```python
from build123d import *

# Parameters (mm, degrees)
F3_R      = 4.7
F4_DEPTH  = 43
F8_DEPTH  = 43
F6_R      = 4.7
F6_R_2    = 4
F9_DEPTH  = 25
F7_R      = 4.7
F7_R_2    = 4
F10_DEPTH = 12
F11_R     = 2.75
F12_DEPTH = 4.701


# Not quite as in the source:
# - ends of sketch curves that miss each other by under 0.0002 mm in the source are joined


with BuildPart() as f4:
    # F3 (on Front) → F4 (new body)
    with BuildSketch(Plane.XZ):
        Circle(F3_R)
    extrude(amount=F4_DEPTH)

    # F5 (on face) → F8 (cut, through all)
    with BuildSketch(Plane.XZ.offset(43)):
        with BuildLine():
            Line((-1.25, -3.8), (0, -3.8))
            Line((0, -3.8), (1.25, -3.8))
            Line((1.25, -3.8), (1.25, -3.7))
            ThreePointArc((1.25, -3.7), (1.3085786438, -3.5585786438), (1.45, -3.5))
            Line((1.45, -3.5), (2, -3.5))
            Line((2, -3.5), (2, -3.05))
            ThreePointArc((2, -3.05), (2.0585786438, -2.9085786438), (2.2, -2.85))
            Line((2.2, -2.85), (3.15, -2.85))
            Line((3.15, -2.85), (3.15, -2.15))
            Line((3.15, -2.15), (2.2, -2.15))
            ThreePointArc((2.2, -2.15), (2.0585786438, -2.0914213562), (2, -1.95))
            Line((2, -1.95), (2, -1.887459))
            ThreePointArc((2, -1.887459), (2.1033535752, -1.771554046), (2.2, -1.65))
            Line((2.2, -1.65), (3.75, -1.65))
            Line((3.75, -1.65), (3.75, 0))
            Line((3.75, 0), (3.75, 1.65))
            Line((3.75, 1.65), (2.2, 1.65))
            ThreePointArc((2.2, 1.65), (2.1033535752, 1.771554046), (1.9999998047, 1.8874588157))
            Line((1.9999998047, 1.8874588157), (2, 1.95))
            ThreePointArc((2, 1.95), (2.0585786438, 2.0914213562), (2.2, 2.15))
            Line((2.2, 2.15), (3.15, 2.15))
            Line((3.15, 2.15), (3.15, 2.85))
            Line((3.15, 2.85), (2.2, 2.85))
            ThreePointArc((2.2, 2.85), (2.0585786438, 2.9085786438), (2, 3.05))
            Line((2, 3.05), (2, 3.5))
            Line((2, 3.5), (1.45, 3.5))
            ThreePointArc((1.45, 3.5), (1.3085786438, 3.5585786438), (1.25, 3.7))
            Line((1.25, 3.7), (1.25, 3.8))
            Line((1.25, 3.8), (0, 3.8))
            Line((0, 3.8), (-1.25, 3.8))
            Line((-1.25, 3.8), (-1.25, 3.7))
            ThreePointArc((-1.25, 3.7), (-1.3085786438, 3.5585786438), (-1.45, 3.5))
            Line((-1.45, 3.5), (-2, 3.5))
            Line((-2, 3.5), (-2, 3.05))
            ThreePointArc((-2, 3.05), (-2.0585786438, 2.9085786438), (-2.2, 2.85))
            Line((-2.2, 2.85), (-3.15, 2.85))
            Line((-3.15, 2.85), (-3.15, 2.15))
            Line((-3.15, 2.15), (-2.2, 2.15))
            ThreePointArc((-2.2, 2.15), (-2.0585786438, 2.0914213562), (-2, 1.95))
            Line((-2, 1.95), (-2, 1.887459))
            ThreePointArc((-2, 1.887459), (-2.1033535752, 1.771554046), (-2.2, 1.65))
            Line((-2.2, 1.65), (-3.75, 1.65))
            Line((-3.75, 1.65), (-3.75, 0))
            Line((-3.75, 0), (-3.75, -1.65))
            Line((-3.75, -1.65), (-2.2, -1.65))
            ThreePointArc((-2.2, -1.65), (-2.1033535752, -1.771554046), (-1.9999998047, -1.8874588157))
            Line((-1.9999998047, -1.8874588157), (-2, -1.95))
            ThreePointArc((-2, -1.95), (-2.0585786438, -2.0914213562), (-2.2, -2.15))
            Line((-2.2, -2.15), (-3.15, -2.15))
            Line((-3.15, -2.15), (-3.15, -2.85))
            Line((-3.15, -2.85), (-2.2, -2.85))
            ThreePointArc((-2.2, -2.85), (-2.0585786438, -2.9085786438), (-2, -3.05))
            Line((-2, -3.05), (-2, -3.5))
            Line((-2, -3.5), (-1.45, -3.5))
            ThreePointArc((-1.45, -3.5), (-1.3085786438, -3.5585786438), (-1.25, -3.7))
            Line((-1.25, -3.7), (-1.25, -3.8))
        make_face()
    extrude(amount=-F8_DEPTH, mode=Mode.SUBTRACT)

    # F6 (on face) → F9 (join)
    with BuildSketch(Plane.XZ.offset(43)):
        Circle(F6_R)
        Circle(F6_R_2, mode=Mode.SUBTRACT)
    extrude(amount=F9_DEPTH)

    # F7 (on face) → F10 (join)
    with BuildSketch(Plane(origin=(0, 0, 0), x_dir=(-1, 0, 0), z_dir=(0, 1, 0))):
        Circle(F7_R)
        Circle(F7_R_2, mode=Mode.SUBTRACT)
    extrude(amount=F10_DEPTH)

    # F11 (on Right) → F12 (cut, through all)
    with BuildSketch(Plane.YZ):
        with Locations((-62, 0)):
            Circle(F11_R)
    extrude(amount=-F12_DEPTH, mode=Mode.SUBTRACT)


solid = f4.part
```
The listing builds one solid part. Answer for the finished solid, in the listing's coordinates (mm). A direction names the side the tool comes from. Coordinates: 2 decimals unless noted, no trailing zeros. Write each loop counter-clockwise with the first axis right and the second up, starting at its lowest first coordinate (ties: lowest second). Pieces come first, ordered by that corner, then holes. Notation, with made-up numbers: (-2, -33) - (31, -33) arc R21 cw to (31, -14) - close; hole circle Ø10 at (53, 29.25). An arc over 180 degrees is marked (long way). Return JSON: item names as keys, results as strings. Group by question number.
1. Which of the six approach directions +Z, -Z, +X, -X, +Y, -Y give full straight-line access (tool end or side, diameter ignored) to faces 3 (the cylindrical face through (0.867, 5.916, -3.905)), 4 (the flat face through (0, -22, -3.8)), 5 (the flat face through (3.75, -22, 0)), 6 (the cylindrical face through (3.815, -55.325, 1.201)), 7 (the cylindrical face through (-4.19, -59.38, 0.83))?
2. A cutting plane is placed at A-A, the plane x = 0. Determine the outline of the cut face in (y, z), plus the area to 3 significant figures.
3. Straight lines are drawn through the part: L1, parallel to Z at x = 3.5, y = 6; L2, parallel to X at y = -27.5, z = -2.75; L3, parallel to Z at x = 0, y = 7. For each, find the intervals that lie inside material, in ascending order.
4. A cutting plane is placed at B-B, the plane z = 0. Determine the outline of the cut face in (x, y), plus the area to 3 significant figures.
5. Determine the mould class of faces 1 (the flat face through (-3, -22, 1.65)), 2 (the flat face through (-2, 12, 4)) for opening direction Z: released by +Z, released by -Z, zero draft, split by the parting line, or undercut.
6. Given pin 1 (1 mm diameter, centred on x = 3, y = -25.5, fed in from +Z); pin 2 (4 mm diameter, centred on x = 3, y = -58, fed in from -Z); pin 3 (4 mm diameter, centred on x = 3.5, y = -42.5, fed in from -Z), each flat-ended and moving along its own axis, determine where each tip first touches the part or whether it passes through.
7. A cutting plane is placed at C-C, the plane y = -57. Determine the outline of the cut face in (x, z).
Ans:
{
 "1": {"face 3": "+Y", "face 4": "+Y, -Y", "face 5": "none", "face 6": "-Y", "face 7": "-X"},
 "2": {"outline": "(-68, -4.7) - (12, -4.7) - (12, -4) - (0, -4) - (0, -3.8) - (-43, -3.8) - (-43, -4) - (-68, -4) - close; (-68, 4) - (-43, 4) - (-43, 3.8) - (0, 3.8) - (0, 4) - (12, 4) - (12, 4.7) - (-68, 4.7) - close", "area": "129 mm²"},
 "3": {"L1": "-3.14 to -1.94, 1.94 to 3.14", "L2": "-3.81 to -3.15, 3.15 to 3.81", "L3": "-4.7 to -4, 4 to 4.7"},
 "4": {"outline": "(-4.7, -68) - (-4, -68) - (-4, -64.75) - (-4.7, -64.75) - close; (-4.7, -59.25) - (-4, -59.25) - (-4, -43) - (-3.75, -43) - (-3.75, 0) - (-4, 0) - (-4, 12) - (-4.7, 12) - close; (3.75, -43) - (4, -43) - (4, -68) - (4.7, -68) - (4.7, 12) - (4, 12) - (4, 0) - (3.75, 0) - close", "area": "130 mm²"},
 "5": {"face 1": "undercut", "face 2": "zero draft"},
 "6": {"pin 1": "z = 3.98", "pin 2": "z = -4.59", "pin 3": "z = -4.45"},
 "7": {"outline": "circle Ø9.4 at (0, 0); hole circle Ø8 at (0, 0)"}
}
